```python
from build123d import *

# Parameters (mm, degrees)
SKETCH1_W           = 279.4
SKETCH1_H           = 57.15
BOSS_EXTRUDE1_DEPTH = 6.35
SKETCH3_W           = 24.892
SKETCH3_H           = 8.89
BOSS_EXTRUDE2_DEPTH = 6.35
SKETCH4_W           = 13.208
SKETCH4_H           = 13.208
CUT_EXTRUDE2_DEPTH  = 145.775822308
SKETCH5_W           = 311.517575851
SKETCH5_H           = 2.54
CUT_EXTRUDE3_DEPTH  = 145.775822308
SKETCH6_W           = 279.4
SKETCH6_H           = 12.7
BOSS_EXTRUDE3_DEPTH = 6.35


with BuildPart() as part:
    # Sketch1 → Boss-Extrude1 (new body)
    with BuildSketch(Plane(origin=(0, 0, 0), x_dir=(1, 0, 0), z_dir=(0, 1, 0))):
        Rectangle(SKETCH1_W, SKETCH1_H)
    extrude(amount=BOSS_EXTRUDE1_DEPTH)

    # Sketch3 → Boss-Extrude2 (add)
    with BuildSketch(Plane(origin=(0, 0, 0), x_dir=(1, 0, 0), z_dir=(0, 1, 0))):
        with Locations((-95.25, -33.02)):
            Rectangle(SKETCH3_W, SKETCH3_H)
        with Locations((-57.15, -33.02)):
            Rectangle(SKETCH3_W, SKETCH3_H)
        with Locations((-19.05, -33.02)):
            Rectangle(SKETCH3_W, SKETCH3_H)
        with Locations((19.05, -33.02)):
            Rectangle(SKETCH3_W, SKETCH3_H)
        with Locations((57.15, -33.02)):
            Rectangle(SKETCH3_W, SKETCH3_H)
        with Locations((95.25, -33.02)):
            Rectangle(SKETCH3_W, SKETCH3_H)
    extrude(amount=BOSS_EXTRUDE2_DEPTH)

    # Sketch4 → Cut-Extrude2 (cut, through all)
    with BuildSketch(Plane(origin=(0, 0, 0), x_dir=(1, 0, 0), z_dir=(0, 1, 0))):
        with Locations((-139.7, 9.525)):
            Rectangle(SKETCH4_W, SKETCH4_H)
        with Locations((-139.7, -15.875)):
            Rectangle(SKETCH4_W, SKETCH4_H)
        with Locations((139.7, -15.875)):
            Rectangle(SKETCH4_W, SKETCH4_H)
        with Locations((139.7, 9.525)):
            Rectangle(SKETCH4_W, SKETCH4_H)
    extrude(amount=CUT_EXTRUDE2_DEPTH, mode=Mode.SUBTRACT)

    # Sketch5 → Cut-Extrude3 (cut, through all)
    with BuildSketch(Plane(origin=(0, 6.35, 0), x_dir=(1, 0, 0), z_dir=(0, 1, 0))):
        with Locations((16.058787925, 27.305)):
            Rectangle(SKETCH5_W, SKETCH5_H)
    extrude(amount=-CUT_EXTRUDE3_DEPTH, mode=Mode.SUBTRACT)

    # Sketch6 → Boss-Extrude3 (add)
    with BuildSketch(Plane(origin=(0, 6.35, 0), x_dir=(1, 0, 0), z_dir=(0, 1, 0))):
        with Locations((0, 32.385)):
            Rectangle(SKETCH6_W, SKETCH6_H)
    extrude(amount=-BOSS_EXTRUDE3_DEPTH)


solid = part.part
```
Geometry: final body of the model. Coordinates: model frame, mm. A direction names the side the tool comes from. Round coordinates to 2 decimals unless told otherwise and drop trailing zeros. Write each loop counter-clockwise with the first axis right and the second up, starting at its lowest first coordinate (ties: lowest second). Pieces come first, ordered by that corner, then holes. Notation, with made-up numbers: M 20.25,70 L 32.25,70 A29 cw 32.25,107 Z; hole C 9,64 d5. An arc over 180 degrees is marked long. Answer in a Markdown table with one row per item. Add a question column.
(1) Draft query along Z for faces 6 (the face through (38, 3, 28.575)), 7 (the face through (-139.7, 3, -27)), 8 (the face through (-136, 3, 9.271)), 9 (the face through (136, 3, -2.921)). Return one class per face: pulls with the +Z half, pulls with the -Z half, needs draft (parallel to the pull), parting line crosses it, or undercut.
(2) Reachability of faces 1 (the face through (6.604, 3, 33)), 2 (the face through (-139.7, 3, 3)), 3 (the face through (123, 3, 28.575)), 4 (the face through (-136, 3, 22.479)), 5 (the face through (-95, 3, 37.465)) from +Z, -Z, +X, -X, +Y, -Y: full face, straight path, thin tool, end or side. Return the list, or none.
(3) Contact query for flat-ended pins moving along their axis: pin 1 (2 mm diameter, centred on y = 1, z = -6, fed in from +X); pin 2 (1.9 mm diameter, centred on y = 2, z = 33, fed in from -X); pin 3 (2 mm diameter, centred on x = 35.5, y = 1.5, fed in from +Z) (3 decimals). Output: stop coordinate, or through.
(4) Cut plane A-A, the plane x = -110.5. Return the cut outline in (y, z) (3 decimals), then the cut area to 3 significant figures.
(5) Ray query, L1, parallel to X at y = 2.5, z = 11.5; L2, parallel to Z at x = -34, y = 0.5 (3 decimals). Return the intervals inside material, ascending.
(6) Cut plane B-B, the plane z = 16. Return the cut outline in (x, y).
Established:
| question | item | result |
|---|---|---|
| 1 | face 6 | pulls with the +Z half |
| 1 | face 7 | needs draft |
| 1 | face 8 | undercut |
| 1 | face 9 | undercut |
| 2 | face 1 | +Z, +Y, -Y |
| 2 | face 2 | +Z, -Z, -X, +Y, -Y |
| 2 | face 3 | +Z, +X, +Y, -Y |
| 2 | face 4 | -X, +Y, -Y |
| 2 | face 5 | +Z, +X, -X, +Y, -Y |
| 3 | pin 1 | x = 133.1 |
| 3 | pin 2 | x = -107.7 |
| 3 | pin 3 | z = 28.575 |
| 4 | outline | M 0,-38.735 L 6.35,-38.735 L 6.35,28.575 L 0,28.575 Z |
| 4 | area | 427 mm² |
| 5 | L1 | -133.1 to 133.1 |
| 5 | L2 | -38.735 to 28.575 |
| 6 | outline | M -133.1,0 L 133.1,0 L 133.1,6.35 L -133.1,6.35 Z |
